Autodesk Inventor part; units mm, degrees
ref_plane "YZ Plane" through (0, 0, 0) normal (1, 0, 0) x (0, 1, 0)
ref_plane "XZ Plane" through (0, 0, 0) normal (0, 1, 0) x (-1, 0, 0)
ref_plane "XY Plane" through (0, 0, 0) normal (0, 0, 1) x (1, 0, 0)
sketch "Sketch1" plane through (0, 0, 0) normal (0, 1, 0) x (-1, 0, 0)
  circle A0 centre (29.5808, -39.6651) radius 1.75
  circle A1 centre (-29.5808, 39.6651) radius 1.75
  circle A2 centre (29.5808, 39.6651) radius 1.75
  circle A3 centre (-29.5808, -39.6651) radius 1.75
  line L0 (-27, -45) -> (27, -45)
  arc A4 (27, -45) -> (35, -37) centre (27, -37) ccw
  line L1 (35, -37) -> (35, 36.8048)
  ellipse E0 centre (27, 36.8048) end of major axis (27, 45) minor radius 8 (35, 36.8048) -> (27, 45) ccw
  line L2 (27, 45) -> (-27, 45)
  ellipse E1 centre (-27, 36.8048) end of major axis (-27, 45) minor radius 8 (-27, 45) -> (-35, 36.8048) ccw
  line L3 (-35, 36.8048) -> (-35, -37)
  arc A5 (-35, -37) -> (-27, -45) centre (-27, -37) ccw
  line L4 (22.5, -42.5) -> (-22.5, -42.5)
  arc A6 (-24.2843, -42.3395) -> (-22.5, -42.5) centre (-22.5, -32.5) ccw
  arc A7 (-24.2843, -42.3395) -> (-32.4877, -32.9952) centre (-33.2764, -41.9606) ccw
  arc A8 (-32.5, -32.5) -> (-32.4877, -32.9952) centre (-22.5, -32.5) ccw
  line L5 (-32.5, -32.5) -> (-32.5, 32.2561)
  ellipse E2 centre (-22.5, 32.2561) end of major axis (-22.5, 42.5) minor radius 10 (-32.4132, 33.603) -> (-32.5, 32.2561) ccw
  arc A9 (-32.4132, 33.603) -> (-23.6584, 42.431) centre (-32.6569, 42.5997) ccw
  ellipse E3 centre (-22.5, 32.2561) end of major axis (-22.5, 42.5) minor radius 10 (-22.5, 42.5) -> (-23.6584, 42.431) ccw
  line L6 (-22.5, 42.5) -> (22.5, 42.5)
  ellipse E4 centre (22.5, 32.2561) end of major axis (22.5, 42.5) minor radius 10 (23.6584, 42.431) -> (22.5, 42.5) ccw
  arc A10 (23.6584, 42.431) -> (32.4132, 33.603) centre (32.6569, 42.5997) ccw
  ellipse E5 centre (22.5, 32.2561) end of major axis (22.5, 42.5) minor radius 10 (32.5, 32.2561) -> (32.4132, 33.603) ccw
  line L7 (32.5, 32.2561) -> (32.5, -32.5)
  arc A11 (32.4877, -32.9952) -> (32.5, -32.5) centre (22.5, -32.5) ccw
  arc A12 (32.4877, -32.9952) -> (24.2843, -42.3395) centre (33.2764, -41.9606) ccw
  arc A13 (22.5, -42.5) -> (24.2843, -42.3395) centre (22.5, -32.5) ccw
  line L8 (-19.7694, -45) -> (13.1764, -45)
  point P0 (0, 0)
  point P1 (0, 0)
extrude "Extrusion1" add sketch "Sketch1" along normal blind 2.2 contours A5 L3 E1 L2 E0 L1 A4 L0 | L4 A6 A7 A8 L5 E2 A9 E3 L6 E4 A10 E5 L7 A11 A12 A13
sketch "Sketch2" plane through (0, 2.2, 0) normal (0, 1, 0) x (1, 0, 0)
  line L0 (27, 45) -> (-27, 45)
  circle A0 centre (-25, 27) radius 1.25
  circle A1 centre (-25, 27) radius 3
  circle A2 centre (25, 27) radius 3
  circle A3 centre (25, 27) radius 1.25
  circle A4 centre (25, -33) radius 3
  circle A5 centre (25, -33) radius 1.25
  circle A6 centre (-25, -33) radius 3
  circle A7 centre (-25, -33) radius 1.25
  line L1 (-27, -45) -> (27, -45)
  point P0 (0, 0)
  point P1 (0, 0)
  point P2 (0, -5)
  dimension "d5" = 2.5
  dimension "d6" = 6
  dimension "d7" = 2.5
  dimension "d8" = 6
  dimension "d9" = 2.5
  dimension "d10" = 6
  dimension "d11" = 2.5
  dimension "d12" = 6
  dimension "d21" = 12
  dimension "d22" = 12
  dimension "d23" = 18
  dimension "d24" = 18
extrude "Extrusion2" add sketch "Sketch2" along normal blind 5
chamfer "Chamfer1" distance 2 angle 45 4 edges at (-28, 2.2, 33) (22, 2.2, 33) (-28, 2.2, -27) (22, 2.2, -27)
properties part number "obudowa - budzik v4 dol dol"
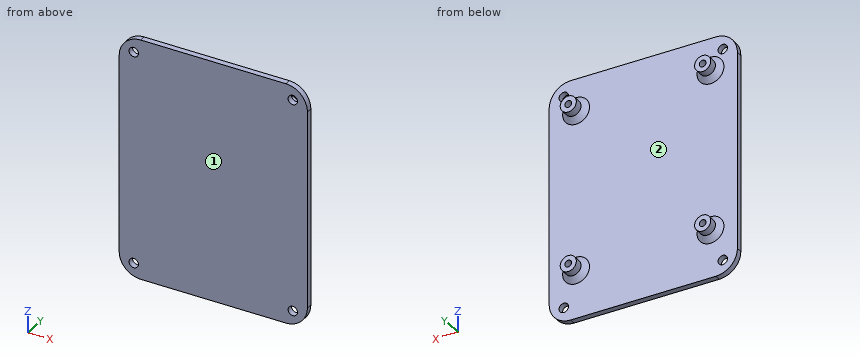
Here's how the part is built. I have some questions about the finished solid (model axes, mm). Face numbers are marked on the shaded views. Give positions to 0.01 mm unless a question says otherwise; leave off trailing zeros. Loops run counter-clockwise (first coordinate to the right, second up) from the corner with the lowest first, then second, coordinate; pieces in that order, holes last. Notation, with made-up numbers: M 68,65 L 113,65 A15 ccw 113,69 Z; hole C -36,51 d11. An arc over 180 degrees is marked long. Put each result on its own line as item: value. Start each with the question number.
(1) If we mould it in two halves opening along X, with no side actions, what happens to the marked faces 1 and 2? For each: +X half, -X half, draft (parallel to the pull), parting line (faces both ways), or undercut.
(2) I want a section at A-A on z = -27. Please give me the cut outline in (x, y).
(3) I need wall thicknesses on line 1 along X through (y, z) = (5.2, 33); line 2 along Z through (x, y) = (-25, 4.5); line 3 along X through (y, z) = (3, 32). Which ranges of each line are inside material? Lowest first, please. Write a range as [from, to].
(4) I want a section at B-B on x = 25. Please give me the cut outline in (y, z).
(5) Will this pin go through, and if not, where does the flat tip stop? pin 1 Ø5.5 at (x, z) = (-29.58, -39.67) entering from +Y.
(6) I want a section at C-C on x = 9. Please give me the cut outline in (y, z).
Answer block:
1. face 1: draft
1. face 2: undercut
2. outline: M -35,0 L 35,0 L 35,2.2 L 30,2.2 L 28,4.2 L 28,7.2 L 26.25,7.2 L 26.25,2.2 L 23.75,2.2 L 23.75,7.2 L 22,7.2 L 22,4.2 L 20,2.2 L -20,2.2 L -22,4.2 L -22,7.2 L -23.75,7.2 L -23.75,2.2 L -26.25,2.2 L -26.25,7.2 L -28,7.2 L -28,4.2 L -30,2.2 L -35,2.2 Z
3. line 1: [-28, -26.25], [-23.75, -22], [22, 23.75], [26.25, 28]
3. line 2: [-30, -28.25], [-25.75, -24], [30, 31.75], [34.25, 36]
3. line 3: [-29.08, -25.75], [-24.25, -20.92], [20.92, 24.25], [25.75, 29.08]
4. outline: M 0,-45 L 2.2,-45 L 2.2,-32 L 4.2,-30 L 7.2,-30 L 7.2,-28.25 L 2.2,-28.25 L 2.2,-25.75 L 7.2,-25.75 L 7.2,-24 L 4.2,-24 L 2.2,-22 L 2.2,28 L 4.2,30 L 7.2,30 L 7.2,31.75 L 2.2,31.75 L 2.2,34.25 L 7.2,34.25 L 7.2,36 L 4.2,36 L 2.2,38 L 2.2,45 L 0,45 Z
5. pin 1: y = 2.2
6. outline: M 0,-45 L 2.2,-45 L 2.2,45 L 0,45 Z
